The listing builds one solid part. Answer for the finished solid, in the listing's coordinates (mm). Round coordinates to 2 decimals unless told otherwise and drop trailing zeros. Order: outer loops, then holes, each group sorted by start corner. A loop starts at its lowest first (then second) coordinate and runs counter-clockwise, first axis right, second up. Notation, with made-up numbers: M 5.25,-4 L 50.25,-4 A26 cw 50.25,32 Z; hole C -30,-18 d5. An arc over 180 degrees is marked long. Write item = value, one per line. Start each with the question number.
(1) Straight lines are drawn through the part: probe 1 along Y at (x, z) = (42.15, 0); probe 2 along Z at (x, y) = (34.5, 17.75); probe 3 along Y at (x, z) = (37.5, 1.25). For each, find the intervals that lie inside material, in ascending order. Write a range as from..to.
(2) Each of these flat-tipped pins is pushed along its axis until it touches: pin 1 (12 mm diameter, centred on y = 19, z = 8, fed in from +X); pin 2 (1 mm diameter, centred on x = 25, z = -3.5, fed in from +Y); pin 3 (3 mm diameter, centred on x = 28, y = 7, fed in from +Z). Where does it stop, or does it pass through?
(3) A cutting plane is placed at B-B, the plane y = 12. Determine the outline of the cut face in (x, z) (3 decimals).
(4) A cutting plane is placed at A-A, the plane z = 0. Determine the outline of the cut face in (x, y) (3 decimals), and give its area (3 significant figures).
(5) A cutting plane is placed at C-C, the plane x = 29.5. Determine the outline of the cut face in (y, z).
from build123d import *
from build123d.topology import SkipClean

# Parameters (mm, degrees)
SKETCH1_R                = 42.725
SKETCH1_R_2              = 15.875
BOSS_EXTRUDE1_DEPTH      = 1
SKETCH2_R                = 42.725
SKETCH2_R_2              = 41.725
SKETCH2_R_3              = 16.875
SKETCH2_R_4              = 15.875
BOSS_EXTRUDE2_DEPTH      = 25
SKETCH3_R                = 9.53
CUT_EXTRUDE1_DEPTH       = 66.778805477
BOSS_EXTRUDE3_REACH      = 67.779
BOSS_EXTRUDE3_END_RADIUS = 42.725
SKETCH9_R                = 11.53
SKETCH9_R_2              = 9.53
CUT_EXTRUDE2_START       = -26.530000265
CUT_EXTRUDE2_DEPTH       = 26.530000265
CUT_EXTRUDE4_DEPTH       = 53.44997753
CUT_EXTRUDE4_DEPTH_BACK  = 53.44997753
SKETCH11_R               = 50
SKETCH11_R_2             = 11.53


# Read off the part's stored shape, not the designer's step: Cut-Extrude2
with BuildPart() as part:
    # Sketch1 → Boss-Extrude1 (new body)
    with BuildSketch(Plane(origin=(0, 0, 0), x_dir=(1, 0, 0), z_dir=(0, 1, 0))):
        with Locations(Location((0, 0, 0), (0, 0, 270))):
            Circle(SKETCH1_R)
        with Locations(Location((0, 0, 0), (0, 0, 270))):
            Circle(SKETCH1_R_2, mode=Mode.SUBTRACT)
    extrude(amount=BOSS_EXTRUDE1_DEPTH)

    # Sketch2 → Boss-Extrude2 (add)
    # profile 1 of 2: a face of its own
    with BuildSketch(Plane(origin=(0, 1, 0), x_dir=(1, 0, 0), z_dir=(0, 1, 0))):
        with Locations(Location((0, 0, 0), (0, 0, 270))):
            Circle(SKETCH2_R)
        with Locations(Location((0, 0, 0), (0, 0, 270))):
            Circle(SKETCH2_R_2, mode=Mode.SUBTRACT)
    # profile 2 of 2: a face of its own
    with BuildSketch(Plane(origin=(0, 1, 0), x_dir=(1, 0, 0), z_dir=(0, 1, 0))):
        with Locations(Location((0, 0, 0), (0, 0, 270))):
            Circle(SKETCH2_R_3)
        with Locations(Location((0, 0, 0), (0, 0, 270))):
            Circle(SKETCH2_R_4, mode=Mode.SUBTRACT)
    extrude(amount=BOSS_EXTRUDE2_DEPTH)

    # Sketch3 → Cut-Extrude1 (cut, through all)
    with BuildSketch(Plane(origin=(0, 0, 0), x_dir=(0, 0, -1), z_dir=(1, 0, 0))):
        with Locations(Location((0, 11, 0), (0, 0, 180))):
            Circle(SKETCH3_R)
    extrude(amount=CUT_EXTRUDE1_DEPTH, mode=Mode.SUBTRACT)

    # Boss-Extrude3: up to this cylinder (the profile starts inside it)
    boss_extrude3_end = Plane(origin=(0, 21.688873, 0), z_dir=(0, -1, 0)) * Cylinder(BOSS_EXTRUDE3_END_RADIUS, 222.008, mode=Mode.PRIVATE)
    # Sketch9 → Boss-Extrude3 (add, up to the surface)
    with BuildSketch(Plane(origin=(0, 0, 0), x_dir=(0, 0, -1), z_dir=(1, 0, 0)), mode=Mode.PRIVATE) as boss_extrude3_sk1:
        with Locations(Location((0, 11, 0), (0, 0, 252.560311876))):
            Circle(SKETCH9_R)
        with Locations(Location((0, 11, 0), (0, 0, 270))):
            Circle(SKETCH9_R_2, mode=Mode.SUBTRACT)
    boss_extrude3_tool1 = extrude(boss_extrude3_sk1.sketch, amount=BOSS_EXTRUDE3_REACH, mode=Mode.PRIVATE) & boss_extrude3_end
    add(boss_extrude3_tool1.solids().sort_by_distance((0, 21.688873, -3.357823))[0])

    # Cut-Extrude2 outline → Cut-Extrude2 (cut)
    with BuildSketch(Plane(origin=(0, 26, 0), x_dir=(1, 0, 0), z_dir=(0, 1, 0)).offset(CUT_EXTRUDE2_START)):
        with BuildLine():
            ThreePointArc((1.562409729, -15.797927106), (15.875, 0), (1.562409729, 15.797927106))
            Line((1.562409729, 15.797927106), (41.036063238, 11.893995921))
            ThreePointArc((41.036063238, 11.893995921), (-42.725, 0), (41.036063238, -11.893995921))
            Line((41.036063238, -11.893995921), (1.562409729, -15.797927106))
        make_face()
    extrude(amount=CUT_EXTRUDE2_DEPTH, mode=Mode.SUBTRACT)

    # Sketch11 → Cut-Extrude4 (cut, two sides: drawn at the far end of the back side and taken through both)
    with SkipClean():  # the faces are left unmerged after this step: merging them gives an invalid solid
        with BuildSketch(Plane(origin=(0, 0, 0), x_dir=(0, 0, -1), z_dir=(1, 0, 0)).offset(-CUT_EXTRUDE4_DEPTH_BACK)):
            with Locations((0, 11)):
                Circle(SKETCH11_R)
            with Locations(Location((0, 11, 0), (0, 0, 180))):
                Circle(SKETCH11_R_2, mode=Mode.SUBTRACT)
        extrude(amount=CUT_EXTRUDE4_DEPTH + CUT_EXTRUDE4_DEPTH_BACK, mode=Mode.SUBTRACT)


solid = part.part
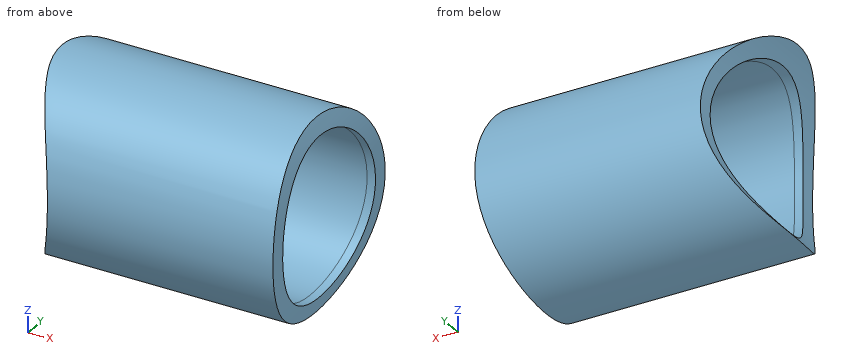
Reported:
q1.probe_1 = -0.53..1.47, 20.53..22.53
q1.probe_2 = -9.35..-6.73, 6.73..9.35
q1.probe_3 = -0.46..1.55, 20.45..22.46
q2.pin_1 = 42.67
q2.pin_2 = 22.13
q2.pin_3 = 11.26
q3.outline = M 10.958,-11.487 L 41.152,-11.487 A42.725 ccw 41.661,-9.477 L 12.736,-9.477 A15.875 cw Z; M 10.958,11.487 A15.875 cw 12.736,9.477 L 41.661,9.477 A42.725 ccw 41.152,11.487 Z
q4.outline = M 15.875,-0.53 L 42.725,-0.53 L 42.725,1.47 L 15.875,1.47 Z; M 15.875,20.53 L 42.725,20.53 L 42.725,22.53 L 15.875,22.53 Z
q4.area = 107 mm²
q5.outline = C 11,0 d23.06; hole C 11,0 d19.06
